from build123d import *

# Parameters (mm, degrees)
SKETCH1_R                           = 6
BOSS_EXTRUDE1_DEPTH                 = 433.48108
CHAMFER1_SIZE                       = 0.5
M5X0_8_TAPPED_HOLE1_D               = 4.2
M5X0_8_TAPPED_HOLE1_DEPTH           = 16.4
M5X0_8_TAPPED_HOLE1_TIP             = 1.2618073
M5X0_8_TAPPED_HOLE1_ON_FACE_2_D     = 4.2
M5X0_8_TAPPED_HOLE1_ON_FACE_2_DEPTH = 16.4
M5X0_8_TAPPED_HOLE1_ON_FACE_2_TIP   = 1.2618073


with BuildPart() as part:
    # Sketch1 → Boss-Extrude1 (new body)
    with BuildSketch(Plane.XY):
        Circle(SKETCH1_R)
    extrude(amount=BOSS_EXTRUDE1_DEPTH)

    # Chamfer1
    chamfer1_edges = [part.edges().sort_by_distance(p)[0] for p in [
        (-6, 0, 0),
        (-6, 0, 433.48108),
    ]]
    chamfer(chamfer1_edges, length=CHAMFER1_SIZE)

    # M5x0.8 Tapped Hole1
    with Locations(Plane(origin=(0, 0, 433.48108), x_dir=(0, 1, 0), z_dir=(0, 0, 1))):
        with Locations((0, 0)):
            Hole(M5X0_8_TAPPED_HOLE1_D / 2, depth=M5X0_8_TAPPED_HOLE1_DEPTH)
            with Locations((0, 0, -(M5X0_8_TAPPED_HOLE1_DEPTH + M5X0_8_TAPPED_HOLE1_TIP / 2))):  # 118° drill point
                Cone(0, M5X0_8_TAPPED_HOLE1_D / 2, M5X0_8_TAPPED_HOLE1_TIP, mode=Mode.SUBTRACT)

    # M5x0.8 Tapped Hole1 on face 2
    with Locations(Plane(origin=(0, 0, 0), x_dir=(-1, 0, 0), z_dir=(0, 0, -1))):
        with Locations((0, 0)):
            Hole(M5X0_8_TAPPED_HOLE1_ON_FACE_2_D / 2, depth=M5X0_8_TAPPED_HOLE1_ON_FACE_2_DEPTH)
            with Locations((0, 0, -(M5X0_8_TAPPED_HOLE1_ON_FACE_2_DEPTH + M5X0_8_TAPPED_HOLE1_ON_FACE_2_TIP / 2))):  # 118° drill point
                Cone(0, M5X0_8_TAPPED_HOLE1_ON_FACE_2_D / 2, M5X0_8_TAPPED_HOLE1_ON_FACE_2_TIP, mode=Mode.SUBTRACT)


solid = part.part
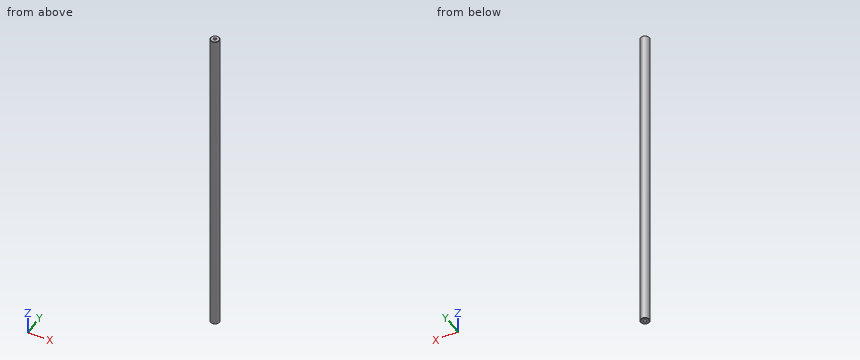
Read the model definition and answer for the solid it produces. Units are mm, in the model's axes. Give positions to 0.01 mm unless a question says otherwise; leave off trailing zeros. Write each loop counter-clockwise with the first axis right and the second up, starting at its lowest first coordinate (ties: lowest second). Pieces come first, ordered by that corner, then holes. Notation, with made-up numbers: (50.25, -5.5) - (96.25, -5.5) arc R17 cw to (96.25, 7.5) - close; hole circle Ø1 at (57, 55). An arc over 180 degrees is marked (long way). Return JSON: item names as keys, results as strings.
Q1. Given P1, Ø4, axis at x = 0, y = 0, coming from the -Z side; P2, Ø6, axis at y = 4, z = 103.5, coming from the +X side, each flat-ended and moving along its own axis, determine where each tip first touches the part or whether it passes through.
Reply:
{"P1": "z = 16.46", "P2": "x = 5.92"}
Q2. A cutting plane is placed at A-A, the plane z = 266.5. Determine the outline of the cut face in (x, y).
Reply:
{"outline": "circle Ø12 at (0, 0)"}
Q3. Consider line 1 along Y through (x, z) = (0, 7); line 2 along Y through (x, z) = (0.25, 160); line 3 along X through (y, z) = (-2.25, 20.5). Determine where each line is inside the solid, lowest interval first. Write a range as [from, to].
Reply:
{"line 1": "[-6, -2.1], [2.1, 6]", "line 2": "[-5.99, 5.99]", "line 3": "[-5.56, 5.56]"}
